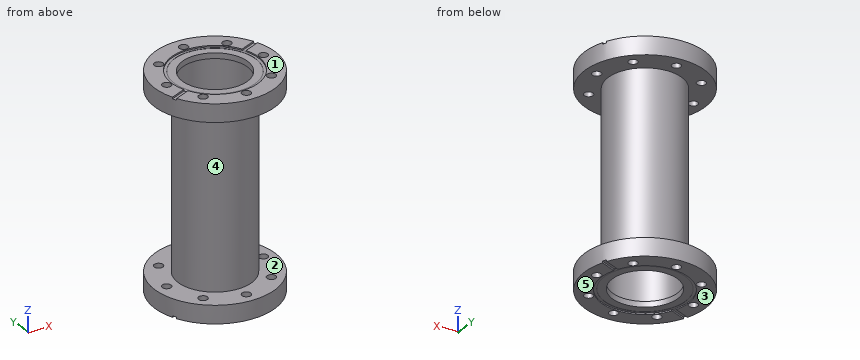
from build123d import *

# Parameters (mm, degrees)
CYLINDER032_R             = 41.25
CYLINDER032_DEPTH         = 1.5
BOX004_W                  = 16.9
BOX004_H                  = 4
BOX004_DEPTH              = 1.5
BOX005_W                  = 16.9
BOX005_H                  = 4
BOX005_DEPTH              = 1.5
FUSION011_PLACEMENT_ANGLE = 22.5
CYLINDER026_R             = 35
CYLINDER026_DEPTH         = 10.6
CYLINDER027_R             = 31
CYLINDER027_DEPTH         = 17
CYLINDER031_R             = 4.2
CYLINDER031_DEPTH         = 17
ARRAY005_COUNT            = 8
CYLINDER030_R             = 38.6
CYLINDER030_DEPTH         = 0.22
CYLINDER029_R             = 41.25
CYLINDER029_DEPTH         = 1.2
CYLINDER028_R             = 57.15
CYLINDER028_DEPTH         = 17
CUT030_PLACEMENT_ANGLE    = 180
COMPOUND_PLACEMENT_ANGLE  = 45
TUBE_R                    = 35
TUBE_R_2                  = 33
TUBE_DEPTH                = 187.2
CYLINDER025_R             = 41.25
CYLINDER025_DEPTH         = 1.5
BOX002_W                  = 16.9
BOX002_H                  = 4
BOX002_DEPTH              = 1.5
BOX003_W                  = 16.9
BOX003_H                  = 4
BOX003_DEPTH              = 1.5
FUSION008_PLACEMENT_ANGLE = 22.5
CYLINDER018_R             = 35
CYLINDER018_DEPTH         = 10.6
CYLINDER019_R             = 31
CYLINDER019_DEPTH         = 17
CYLINDER023_R             = 4.2
CYLINDER023_DEPTH         = 17
ARRAY004_COUNT            = 8
CYLINDER022_R             = 38.6
CYLINDER022_DEPTH         = 0.22
CYLINDER021_R             = 41.25
CYLINDER021_DEPTH         = 1.2
CYLINDER020_R             = 57.15
CYLINDER020_DEPTH         = 17


with BuildPart() as cylinder032:
    # Cylinder032 → Cylinder032 (new body)
    with BuildSketch(Plane.XY):
        Circle(CYLINDER032_R)
    extrude(amount=CYLINDER032_DEPTH)


with BuildPart() as cube004:
    # Box004 → Box004 (new body)
    with BuildSketch(Plane(origin=(40.75, -2, 0), x_dir=(1, 0, 0), z_dir=(0, 0, 1))):
        with Locations((8.45, 2)):
            Rectangle(BOX004_W, BOX004_H)
    extrude(amount=BOX004_DEPTH)


with BuildPart() as obj1:
    # Box005 → Box005 (new body)
    with BuildSketch(Plane(origin=(-57.65, -2, 0), x_dir=(1, 0, 0), z_dir=(0, 0, 1))):
        with Locations((8.45, 2)):
            Rectangle(BOX005_W, BOX005_H)
    extrude(amount=BOX005_DEPTH)

    # Fusion011: union Cube004
    add(cube004.part)


with BuildPart() as obj1_1:
    # Fusion011 placement: moved
    add(obj1.part.rotate(Axis((0, 0, 0), (0, 0, 1)), FUSION011_PLACEMENT_ANGLE))

    # Cut029: cut Cylinder032
    add(cylinder032.part, mode=Mode.SUBTRACT)


with BuildPart() as cylinder026:
    # Cylinder026 → Cylinder026 (new body)
    with BuildSketch(Plane.XY.offset(6.4)):
        Circle(CYLINDER026_R)
    extrude(amount=CYLINDER026_DEPTH)


with BuildPart() as fusion010:
    # Cylinder027 → Cylinder027 (new body)
    with BuildSketch(Plane.XY):
        Circle(CYLINDER027_R)
    extrude(amount=CYLINDER027_DEPTH)

    # Fusion010: union Cylinder026
    add(cylinder026.part)


with BuildPart() as boltholearray005:
    # Cylinder031 → Cylinder031 (new body)
    with BuildSketch(Plane(origin=(46.1, 0, 0), x_dir=(1, 0, 0), z_dir=(0, 0, 1))):
        Circle(CYLINDER031_R)
    extrude(amount=CYLINDER031_DEPTH)

    # Array005: BoltHoleArray005 ×8 about axis
    array005_axis = Axis((0, 0, 0), (0, 0, 1))


with BuildPart() as boltholearray005_1:
    add(boltholearray005.part)
    for i in range(1, ARRAY005_COUNT):
        add(boltholearray005.part.rotate(array005_axis, i * 360 / ARRAY005_COUNT))


with BuildPart() as cylinder030:
    # Cylinder030 → Cylinder030 (new body)
    with BuildSketch(Plane.XY):
        Circle(CYLINDER030_R)
    extrude(amount=CYLINDER030_DEPTH)


with BuildPart() as knifeedge005:
    # Cone005 → Cone005 (revolve)
    with BuildSketch(Plane.XZ):
        Polygon((0, 0), (38.6, 0), (41.25, 0.22), (0, 0.22), align=None)
    revolve(axis=Axis((0, 0, 0), (0, 0, 1)))

    # Cut026: cut Cylinder030
    add(cylinder030.part, mode=Mode.SUBTRACT)


with BuildPart() as knifeedge005_1:
    # Cut026 placement: moved
    add(knifeedge005.part.moved(Location((0, 0, 0.98))))


with BuildPart() as sealrecess005:
    # Cylinder029 → Cylinder029 (new body)
    with BuildSketch(Plane.XY):
        Circle(CYLINDER029_R)
    extrude(amount=CYLINDER029_DEPTH)


with BuildPart() as obj2:
    # Cylinder028 → Cylinder028 (new body)
    with BuildSketch(Plane.XY):
        Circle(CYLINDER028_R)
    extrude(amount=CYLINDER028_DEPTH)

    # Cut025: cut SealRecess005
    add(sealrecess005.part, mode=Mode.SUBTRACT)

    # Fusion009: union KnifeEdge005
    add(knifeedge005_1.part)

    # Cut027: cut BoltHoleArray005
    add(boltholearray005_1.part, mode=Mode.SUBTRACT)

    # Cut028: cut Fusion010
    add(fusion010.part, mode=Mode.SUBTRACT)

    # Cut030: cut obj1
    add(obj1_1.part, mode=Mode.SUBTRACT)


with BuildPart() as obj2_1:
    # Cut030 placement: moved
    add(obj2.part.moved(Location((0, 0, 200))).rotate(Axis((0, 0, 200), (1, 0, 0)), CUT030_PLACEMENT_ANGLE))


with BuildPart() as obj2_2:
    # Compound placement: moved
    add(obj2_1.part.rotate(Axis((0, 0, 0), (0, 0, 1)), COMPOUND_PLACEMENT_ANGLE))


with BuildPart() as tube:
    # Tube → Tube (new body)
    with BuildSketch(Plane.XY.offset(6.4)):
        Circle(TUBE_R)
        Circle(TUBE_R_2, mode=Mode.SUBTRACT)
    extrude(amount=TUBE_DEPTH)


with BuildPart() as cylinder025:
    # Cylinder025 → Cylinder025 (new body)
    with BuildSketch(Plane.XY):
        Circle(CYLINDER025_R)
    extrude(amount=CYLINDER025_DEPTH)


with BuildPart() as cube002:
    # Box002 → Box002 (new body)
    with BuildSketch(Plane(origin=(40.75, -2, 0), x_dir=(1, 0, 0), z_dir=(0, 0, 1))):
        with Locations((8.45, 2)):
            Rectangle(BOX002_W, BOX002_H)
    extrude(amount=BOX002_DEPTH)


with BuildPart() as obj3:
    # Box003 → Box003 (new body)
    with BuildSketch(Plane(origin=(-57.65, -2, 0), x_dir=(1, 0, 0), z_dir=(0, 0, 1))):
        with Locations((8.45, 2)):
            Rectangle(BOX003_W, BOX003_H)
    extrude(amount=BOX003_DEPTH)

    # Fusion008: union Cube002
    add(cube002.part)


with BuildPart() as obj3_1:
    # Fusion008 placement: moved
    add(obj3.part.rotate(Axis((0, 0, 0), (0, 0, 1)), FUSION008_PLACEMENT_ANGLE))

    # Cut021: cut Cylinder025
    add(cylinder025.part, mode=Mode.SUBTRACT)


with BuildPart() as cylinder018:
    # Cylinder018 → Cylinder018 (new body)
    with BuildSketch(Plane.XY.offset(6.4)):
        Circle(CYLINDER018_R)
    extrude(amount=CYLINDER018_DEPTH)


with BuildPart() as fusion006:
    # Cylinder019 → Cylinder019 (new body)
    with BuildSketch(Plane.XY):
        Circle(CYLINDER019_R)
    extrude(amount=CYLINDER019_DEPTH)

    # Fusion006: union Cylinder018
    add(cylinder018.part)


with BuildPart() as boltholearray004:
    # Cylinder023 → Cylinder023 (new body)
    with BuildSketch(Plane(origin=(46.1, 0, 0), x_dir=(1, 0, 0), z_dir=(0, 0, 1))):
        Circle(CYLINDER023_R)
    extrude(amount=CYLINDER023_DEPTH)

    # Array004: BoltHoleArray004 ×8 about axis
    array004_axis = Axis((0, 0, 0), (0, 0, 1))


with BuildPart() as boltholearray004_1:
    add(boltholearray004.part)
    for i in range(1, ARRAY004_COUNT):
        add(boltholearray004.part.rotate(array004_axis, i * 360 / ARRAY004_COUNT))


with BuildPart() as cylinder022:
    # Cylinder022 → Cylinder022 (new body)
    with BuildSketch(Plane.XY):
        Circle(CYLINDER022_R)
    extrude(amount=CYLINDER022_DEPTH)


with BuildPart() as knifeedge004:
    # Cone004 → Cone004 (revolve)
    with BuildSketch(Plane.XZ):
        Polygon((0, 0), (38.6, 0), (41.25, 0.22), (0, 0.22), align=None)
    revolve(axis=Axis((0, 0, 0), (0, 0, 1)))

    # Cut016: cut Cylinder022
    add(cylinder022.part, mode=Mode.SUBTRACT)


with BuildPart() as knifeedge004_1:
    # Cut016 placement: moved
    add(knifeedge004.part.moved(Location((0, 0, 0.98))))


with BuildPart() as sealrecess004:
    # Cylinder021 → Cylinder021 (new body)
    with BuildSketch(Plane.XY):
        Circle(CYLINDER021_R)
    extrude(amount=CYLINDER021_DEPTH)


with BuildPart() as obj4:
    # Cylinder020 → Cylinder020 (new body)
    with BuildSketch(Plane.XY):
        Circle(CYLINDER020_R)
    extrude(amount=CYLINDER020_DEPTH)

    # Cut015: cut SealRecess004
    add(sealrecess004.part, mode=Mode.SUBTRACT)

    # Fusion005: union KnifeEdge004
    add(knifeedge004_1.part)

    # Cut017: cut BoltHoleArray004
    add(boltholearray004_1.part, mode=Mode.SUBTRACT)

    # Cut018: cut Fusion006
    add(fusion006.part, mode=Mode.SUBTRACT)

    # Cut024: cut obj3
    add(obj3_1.part, mode=Mode.SUBTRACT)

    # Fusion: union obj2, Tube
    add(obj2_2.part)
    add(tube.part)


solid = obj4.part
Build history of the part. All positions in model axes, mm. Face numbers are marked on the shaded views. A direction names the side the tool comes from. Give positions to 0.01 mm unless a question says otherwise; leave off trailing zeros. Write each loop counter-clockwise with the first axis right and the second up, starting at its lowest first coordinate (ties: lowest second). Pieces come first, ordered by that corner, then holes. Notation, with made-up numbers: (75, 45.25) - (116, 45.25) arc R38 cw to (116, 84.25) - close; hole circle Ø5 at (82.25, 6.5). An arc over 180 degrees is marked (long way). Use one line per item in the form item = value. Start each with the question number.
1. Band-saw the part on D-D on x = -46.1. Write the cut outline in (y, z).
2. Drop flat-ended pins along their axis: pin 1 Ø6 at (x, z) = (24, 41) entering from +Y; pin 2 Ø2 at (x, z) = (10, 52.5) entering from -Y; pin 3 Ø5 at (y, z) = (24, 117) entering from -X. Give the stop position or say it passes through.
3. Probe line 1 (Z direction, x = -21, y = 48.5); line 2 (X direction, y = 5.5, z = 83); line 3 (Y direction, x = 46.1, z = 188.25). List the from-to ranges inside material, lowest first. Write a range as [from, to].
4. Two-plate mould, pull along Z, no slides. Class the marked faces 1, 2 and 3: released by +Z, released by -Z, zero draft, split by the parting line, or undercut.
5. Band-saw the part on C-C on z = 140.5. Write the cut outline in (x, y).
6. Band-saw the part on B-B on x = 46. Write the cut outline in (y, z).
7. Band-saw the part on A-A on y = 46.1. Write the cut outline in (x, z), plus the area to 3 significant figures.
8. 3-axis set-ups, long thin cutter, end or side, ignore diameter. For the marked faces 4 and 5: which of +Z, -Z, +X, -X, +Y, -Y reach the whole face in a straight line?
Conclusion:
q1.outline = (-33.78, 0) - (-21.26, 0) - (-21.26, 1.5) - (-16.93, 1.5) - (-16.93, 0) - (-4.2, 0) - (-4.2, 17) - (-33.78, 17) - close; (-33.78, 183) - (-4.2, 183) - (-4.2, 200) - (-16.93, 200) - (-16.93, 198.5) - (-21.26, 198.5) - (-21.26, 200) - (-33.78, 200) - close; (4.2, 0) - (33.78, 0) - (33.78, 17) - (4.2, 17) - close; (4.2, 183) - (33.78, 183) - (33.78, 200) - (4.2, 200) - close
q2.pin_1 = 28
q2.pin_2 = -33.82
q2.pin_3 = -27.62
q3.line_1 = [0, 17], [183, 200]
q3.line_2 = [-34.57, -32.54], [32.54, 34.57]
q3.line_3 = [-33.78, -4.2], [4.2, 33.78]
q4.face_1 = released by +Z
q4.face_2 = undercut
q4.face_3 = released by -Z
q5.outline = circle Ø70 at (0, 0); hole circle Ø66 at (0, 0)
q6.outline = (-33.91, 0) - (-4.2, 0) - (-4.2, 17) - (-33.91, 17) - close; (-33.91, 183) - (-4.2, 183) - (-4.2, 200) - (-33.91, 200) - close; (4.2, 0) - (16.89, 0) - (16.89, 1.5) - (21.22, 1.5) - (21.22, 0) - (33.91, 0) - (33.91, 17) - (4.2, 17) - close; (4.2, 183) - (33.91, 183) - (33.91, 200) - (21.22, 200) - (21.22, 198.5) - (16.89, 198.5) - (16.89, 200) - (4.2, 200) - close
q7.outline = (-33.78, 0) - (-4.2, 0) - (-4.2, 17) - (-33.78, 17) - close; (-33.78, 183) - (-4.2, 183) - (-4.2, 200) - (-33.78, 200) - close; (4.2, 0) - (33.78, 0) - (33.78, 17) - (4.2, 17) - close; (4.2, 183) - (33.78, 183) - (33.78, 200) - (4.2, 200) - close
q7.area = 2,010 mm²
q8.face_4 = none
q8.face_5 = -Z, +X, -X, +Y, -Y
